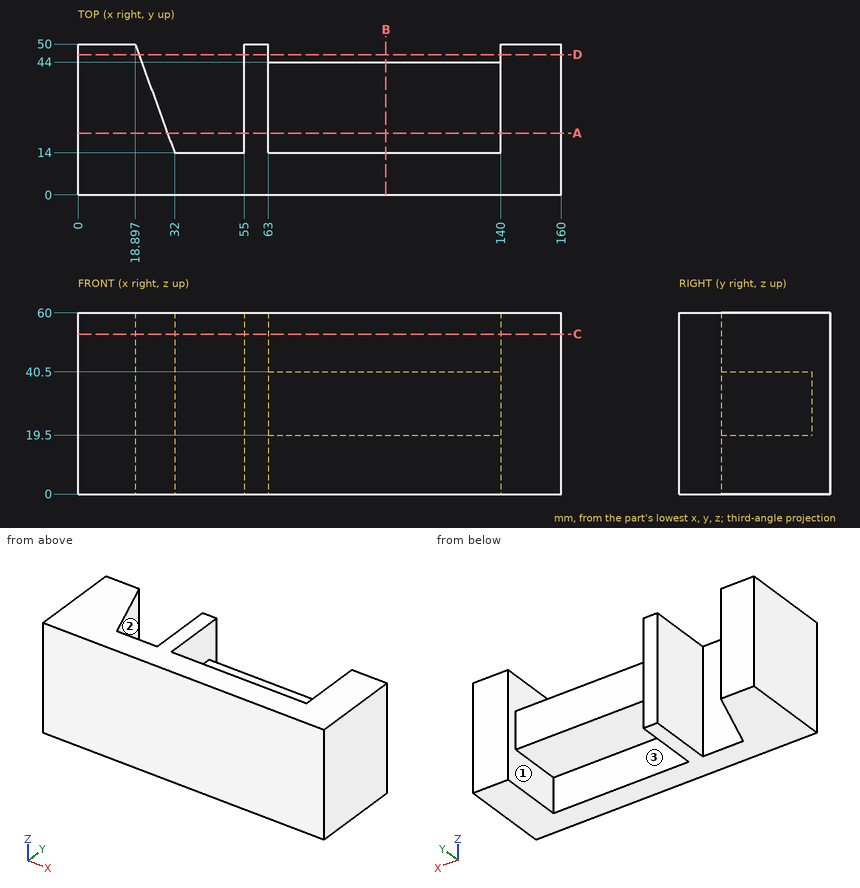
Drawing for the job (mm, zero at the part's lowest x, y, z). A direction names the side the tool comes from. Give positions to 0.01 mm unless a question says otherwise; leave off trailing zeros. Loops run counter-clockwise (first coordinate to the right, second up) from the corner with the lowest first, then second, coordinate; pieces in that order, holes last. Notation, with made-up numbers: M -0.75,7 L 54.25,7 A23 ccw 54.25,33 Z; hole C 74,31 d9. An arc over 180 degrees is marked long. Use one line per item in the form item = value.
Item 1: Slice it at A-A (y = 20.5). List the corners of the cut face in (x, z), plus the area to 4 significant figures.
Determined:
outline = M 0,0 L 29.63,0 L 29.63,60 L 0,60 Z; M 55,0 L 63,0 L 63,19.5 L 140,19.5 L 140,0 L 160,0 L 160,60 L 140,60 L 140,40.5 L 63,40.5 L 63,60 L 55,60 Z
area = 5,075 mm2
Item 2: Slice it at B-B (x = 102). List the corners of the cut face in (y, z), plus the area to 3 significant figures.
Determined:
outline = M 0,0 L 14,0 L 14,19.5 L 44,19.5 L 44,40.5 L 14,40.5 L 14,60 L 0,60 Z
area = 1,470 mm2
Item 3: Slice it at D-D (y = 46.5). List the corners of the cut face in (x, z).
Determined:
outline = M 0,0 L 20.17,0 L 20.17,60 L 0,60 Z; M 55,0 L 63,0 L 63,60 L 55,60 Z; M 140,0 L 160,0 L 160,60 L 140,60 Z
Item 4: Drill centre lines: probe 1 along X at (y, z) = (19, 48.5); probe 2 along X at (y, z) = (25, 6); probe 3 along Y at (x, z) = (117, 14). Where is each one in solid material? Low to high. Write a range as from..to.
Determined:
probe_1 = 0..30.18, 55..63, 140..160
probe_2 = 0..28, 55..63, 140..160
probe_3 = 0..14
Item 5: Slice it at C-C (z = 53). List the corners of the cut face in (x, y).
Determined:
outline = M 0,0 L 160,0 L 160,50 L 140,50 L 140,14 L 63,14 L 63,50 L 55,50 L 55,14 L 32,14 L 18.9,50 L 0,50 Z
Item 6: Flat gauge pins, fed straight in: pin 1 (2 mm diameter, centred on x = 129, y = 22.5, fed in from -Z); pin 2 (12 mm diameter, centred on x = 92.5, z = 53.5, fed in from +Y); pin 3 (6 mm diameter, centred on y = 12.5, z = 7.5, fed in from -X); pin 4 (17 mm diameter, centred on x = 108.5, z = 30, fed in from +Y). Where does each tip first touch, or does it go through?
Determined:
pin_1 = 19.5
pin_2 = 14
pin_3 = 0
pin_4 = 44
Item 7: Which spindle directions (+Z, -Z, +X, -X, +Y, -Y) get a long thin tool onto all of the face, cutting with end or side? Do the marked faces 1, 2 and 3. Say none if no direction does.
Determined:
face_1 = +Y
face_2 = +Z, -Z, +Y
face_3 = -Z, +Y
